Read the model definition and answer for the solid it produces. Units are mm, in the model's axes. Face numbers are marked on the shaded views. Coordinates: 2 decimals unless noted, no trailing zeros. Write each loop counter-clockwise with the first axis right and the second up, starting at its lowest first coordinate (ties: lowest second). Pieces come first, ordered by that corner, then holes. Notation, with made-up numbers: (38, 6.25) -> (72, 6.25) arc R17 cw to (72, 38.25) -> close; hole circle Ø4 at (70.25, 2.25). An arc over 180 degrees is marked (long way). Answer in a Markdown table with one row per item. Add a question column.
Item 1: For a pull along Y with two mould halves and no side action, classify the marked faces 1, 2, 3 and 4 as +Y half, -Y half, draft (parallel to the pull), parting line (faces both ways), or undercut.
Item 2: Section B-B on z = 32 is taken. Count the separate pieces of the cut face and the enclosed holes in it, then the cut area to 3 significant figures.
Item 3: Section C-C on y = 0.5 is taken. Write down the section's boundary in (x, z), then the cut area to 3 significant figures.
Item 4: Straight lines are drawn through the part: line 1 (Y direction, x = -63, z = 36); line 2 (Z direction, x = -68.5, y = 18); line 3 (Y direction, x = -69, z = 20.5). For each, find the intervals that lie inside material, in ascending order. Write a range as from..to.
Item 5: Section A-A on y = -11 is taken. Write down the section's boundary in (x, z), then the cut area to 3 significant figures.
Item 6: Given pin 1 Ø2 at (x, y) = (-47, -13.5) entering from +Z; pin 2 Ø4 at (x, z) = (-65, 49) entering from +Y; pin 3 Ø1 at (x, y) = (-51.5, -19) entering from -Z; pin 4 Ø1.5 at (x, z) = (-46.5, 47.5) entering from +Y, each flat-ended and moving along its own axis, determine where each tip first touches the part or whether it passes through.
```python
from build123d import *

# Parameters (mm, degrees)
BOSS_EXTRUDE1_OUTLINE_R = 2.15
BOSS_EXTRUDE1_DEPTH     = 4.45
BOSS_EXTRUDE2_START     = 1.2515
SKETCH2_R               = 2.15
BOSS_EXTRUDE2_DEPTH     = 4.45
BOSS_EXTRUDE3_DEPTH     = 1.251499962


# Read off the part's stored shape, not the designer's step: Boss-Extrude1
with BuildPart() as part:
    # Boss-Extrude1 outline → Boss-Extrude1 (new body)
    with BuildSketch(Plane(origin=(-50.959815044, -20.804257374, 29.421662933), x_dir=(-0.4364357804719844, -0.17817416127494956, -0.8819171036881971), z_dir=(0.8164965809277264, 0.3333333333333333, -0.4714045207910314))):
        Polygon((-19.487444888, 33.335644756), (5.258463865, 38.097997116), (1.667801371, 56.755626731), (-23.078107381, 51.993274371), align=None)
        with BuildLine():
            ThreePointArc((-14.857414364, 34.568841104), (-17.094425047, 37.205029513), (-15.59724376, 40.32146246))
            Line((-15.59724376, 40.32146246), (-15.535066644, 40.329458894))
            ThreePointArc((-15.535066644, 40.329458894), (-17.069629265, 37.208218432), (-14.795237248, 34.576837538))
            Line((-14.795237248, 34.576837538), (-14.857414364, 34.568841104))
        make_face(mode=Mode.SUBTRACT)
        with Locations((-13.94536077, 37.610022328)):
            Circle(BOSS_EXTRUDE1_OUTLINE_R, mode=Mode.SUBTRACT)
        Polygon((-11.370861729, 47.830728875), (-16.446050654, 40.336567322), (-19.205062219, 39.805595299), (-20.414548532, 46.090270538), align=None, mode=Mode.SUBTRACT)
        with BuildLine():
            Line((-10.795931949, 43.204869293), (-11.349147903, 46.079416754))
            ThreePointArc((-11.349147903, 46.079416754), (-11.103747968, 46.531394654), (-10.775137708, 46.927021304))
            Line((-10.775137708, 46.927021304), (-7.900590246, 47.480237259))
            ThreePointArc((-7.900590246, 47.480237259), (-7.448612347, 47.234837323), (-7.052985696, 46.906227063))
            Line((-7.052985696, 46.906227063), (-6.499769742, 44.031679602))
            ThreePointArc((-6.499769742, 44.031679602), (-6.745169677, 43.579701702), (-7.073779937, 43.184075051))
            Line((-7.073779937, 43.184075051), (-9.948327399, 42.630859097))
            ThreePointArc((-9.948327399, 42.630859097), (-10.400305299, 42.876259032), (-10.795931949, 43.204869293))
        make_face(mode=Mode.SUBTRACT)
        Polygon((-1.422691887, 49.745255053), (1.385418702, 50.285676188), (2.594905016, 44.00100095), (-6.497880812, 42.251093501), align=None, mode=Mode.SUBTRACT)
        with Locations((-3.874282746, 52.481249159)):
            Circle(BOSS_EXTRUDE1_OUTLINE_R, mode=Mode.SUBTRACT)
    extrude(amount=BOSS_EXTRUDE1_DEPTH)


with BuildPart() as body_2:
    # Sketch2 → Boss-Extrude2 (new body)
    with BuildSketch(Plane(origin=(-6.181776854, 0, -10.707151593), x_dir=(-0.866025403784439, 0, 0.4999999999999995), z_dir=(-0.49999999999999944, 0, -0.8660254037844389)).offset(BOSS_EXTRUDE2_START)):
        with BuildLine():
            Line((70.982570609, 13.530711728), (79.145309345, -31.347065587))
            Line((79.145309345, -31.347065587), (58.445309345, -31.347065587))
            ThreePointArc((58.445309345, -31.347065587), (58.677489694, 2.412466855), (73.120403707, 32.927416852))
            Line((73.120403707, 32.927416852), (77.315903942, 31.444083519))
            Line((77.315903942, 31.444083519), (70.982570609, 13.530711728))
        make_face()
        with Locations(Location((62.445309345, -27.347065587, 0), (0, 0, 180))):
            Circle(SKETCH2_R, mode=Mode.SUBTRACT)
        with Locations(Location((62.445309345, -14.647065587, 0), (0, 0, 180))):
            Circle(SKETCH2_R, mode=Mode.SUBTRACT)
        with Locations(Location((75.145309345, -27.347065587, 0), (0, 0, 180))):
            Circle(SKETCH2_R, mode=Mode.SUBTRACT)
    extrude(amount=BOSS_EXTRUDE2_DEPTH)


with BuildPart() as body_3:
    # Sketch4 → Boss-Extrude3 (new body)
    with BuildSketch(Plane(origin=(-6.181776854, 0, -10.707151593), x_dir=(-0.866025403784439, 0, 0.4999999999999995), z_dir=(-0.49999999999999944, 0, -0.8660254037844389))):
        Polygon((70.982570609, 13.530711728), (77.315903942, 31.444083519), (73.120403707, 32.927416852), (66.787070374, 15.014045062), align=None)
    extrude(amount=BOSS_EXTRUDE3_DEPTH)


with BuildPart() as body_4:
    # Mirror1: mirrored copy
    add(body_2.part.mirror(Plane(origin=(0.118223146, 0, 0.204768495), x_dir=(-0.8660254037844389, 0, 0.49999999999999967), z_dir=(0.49999999999999944, 0, 0.8660254037844389))))


with BuildPart() as body_5:
    # Mirror1 2: mirrored copy
    add(body_3.part.mirror(Plane(origin=(0.118223146, 0, 0.204768495), x_dir=(-0.8660254037844389, 0, 0.49999999999999967), z_dir=(0.49999999999999944, 0, 0.8660254037844389))))


with BuildPart() as body_2_1:
    add(body_2.part)

    # Combine1: union body 3, body 4, body 5, part
    add(body_3.part)
    add(body_4.part)
    add(body_5.part)
    add(part.part)


solid = body_2_1.part
```
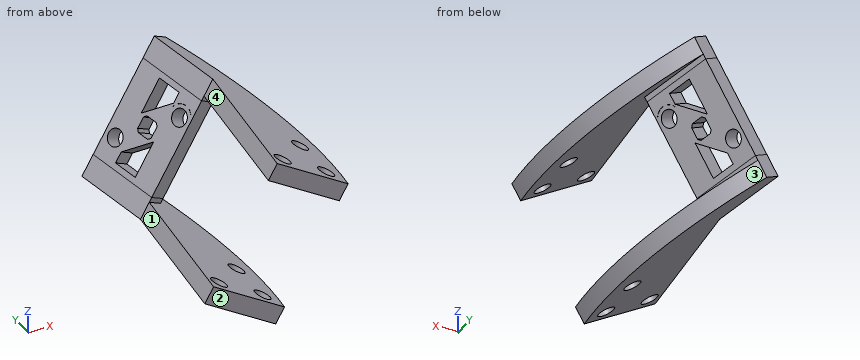
Results below:
| question | item | result |
|---|---|---|
| 1 | face 1 | undercut |
| 1 | face 2 | -Y half |
| 1 | face 3 | parting line |
| 1 | face 4 | undercut |
| 2 | separate pieces | 3 |
| 2 | enclosed holes | 0 |
| 2 | area | 61.8 mm2 |
| 3 | outline | (-72.56, 21.03) -> (-59.49, 13.49) -> (-57.27, 17.34) -> (-70.33, 24.89) -> close; (-56.48, 48.88) -> (-43.42, 41.33) -> (-41.19, 45.19) -> (-54.26, 52.73) -> close |
| 3 | area | 134 mm2 |
| 4 | line 1 | y = 17.99..20.74, 25.38..31.34 |
| 4 | line 2 | z = 18.69..26.48 |
| 4 | line 3 | y = -31.35..28.62 |
| 5 | outline | (-74.37, 22.08) -> (-58.24, 12.76) -> (-56.01, 16.62) -> (-72.14, 25.93) -> close; (-58.29, 49.92) -> (-42.16, 40.61) -> (-39.94, 44.46) -> (-56.07, 53.78) -> close |
| 5 | area | 166 mm2 |
| 6 | pin 1 | stops at z = 49.12 |
| 6 | pin 2 | passes through |
| 6 | pin 3 | stops at z = 45.71 |
| 6 | pin 4 | stops at y = 19.57 |
